```python
from build123d import *

# Parameters (mm, degrees)
F0_W     = 1168.4
F0_H     = 1676.4
F1_DEPTH = 3.175
F2_W     = 1168.4
F2_H     = 3.175
F3_DEPTH = 50.8


# Not quite as in the source:
# - a length typed as a fraction of an inch, garbled in the dataset ("3 / 203.2 mm" for 3/8 in), is restored


with BuildPart() as f1:
    # F0 (on Top) → F1 (new body)
    with BuildSketch(Plane.XY):
        with Locations((-584.2, 838.2)):
            Rectangle(F0_W, F0_H)
    extrude(amount=F1_DEPTH)

    # F2 (on Top) → F3 (join)
    with BuildSketch(Plane.XY):
        Polygon((-1168.4, -3.175), (-1168.4, 0), (-1168.4, 1676.4), (-1168.4, 1679.575), (-1171.575, 1679.575), (-1171.575, -3.175), align=None)
        with Locations((-584.2, 1677.9875)):
            Rectangle(F2_W, F2_H)
        Polygon((0, 1676.4), (0, 0), (0, -3.175), (3.175, -3.175), (3.175, 1679.575), (0, 1679.575), align=None)
        with Locations((-584.2, -1.5875)):
            Rectangle(F2_W, F2_H)
    extrude(amount=F3_DEPTH)


solid = f1.part
```
Design review of the part built by this model. Coordinates are the model's own, in mm. A direction names the side the tool comes from. Coordinates: 2 decimals unless noted, no trailing zeros. Write each loop counter-clockwise with the first axis right and the second up, starting at its lowest first coordinate (ties: lowest second). Pieces come first, ordered by that corner, then holes.
1) Add section B-B (y = 146.5). Write out the cut boundary in (x, z) (3 decimals).
2) Add section A-A (x = -604.5). Write out the cut boundary in (y, z) (3 decimals).
3) Machinability: for faces 1 (the flat face through (-1171.575, 850, 25)), 2 (the flat face through (-592, 850, 3.175)), which of the approach directions +Z, -Z, +X, -X, +Y, -Y give a long, thin tool a straight path to every point of the face, cutting with its end or side? Answer none if there is none.
4) To check wall thickness, follow L1, parallel to X at y = 607, z = 44.5 (3 decimals); L2, parallel to Y at x = -655.5, z = 47 (3 decimals); L3, parallel to Z at x = -68.5, y = 1471 (3 decimals). State the ranges of each line that lie inside material, in increasing order.
5) Mouldability with a two-part tool opening along Y and no side actions: class faces 3 (the flat face through (-592, 1676.4, 27)), 4 (the flat face through (3.175, 826, 25)), 5 (the flat face through (-592, -3.175, 25)) as +Y half, -Y half, draft (parallel to the pull), parting line (faces both ways), or undercut.
6) Add section C-C (z = 21). Write out the cut boundary in (x, y) (3 decimals), plus the area to 3 significant figures.
Check result:
1. outline: (-1171.575, 0) - (3.175, 0) - (3.175, 50.8) - (0, 50.8) - (0, 3.175) - (-1168.4, 3.175) - (-1168.4, 50.8) - (-1171.575, 50.8) - close
2. outline: (-3.175, 0) - (1679.575, 0) - (1679.575, 50.8) - (1676.4, 50.8) - (1676.4, 3.175) - (0, 3.175) - (0, 50.8) - (-3.175, 50.8) - close
3. face 1: +Z, -Z, -X, +Y, -Y
3. face 2: +Z
4. L1: x = -1171.575 to -1168.4, 0 to 3.175
4. L2: y = -3.175 to 0, 1676.4 to 1679.575
4. L3: z = 0 to 3.175
5. face 3: undercut
5. face 4: draft
5. face 5: -Y half
6. outline: (-1171.575, -3.175) - (3.175, -3.175) - (3.175, 1679.575) - (-1171.575, 1679.575) - close; hole (-1168.4, 0) - (0, 0) - (0, 1676.4) - (-1168.4, 1676.4) - close
6. area: 18,100 mm2
